Geometry: final body of the model. Coordinates: model frame, mm. A direction names the side the tool comes from. Give positions to 0.01 mm unless a question says otherwise; leave off trailing zeros. Loops run counter-clockwise (first coordinate to the right, second up) from the corner with the lowest first, then second, coordinate; pieces in that order, holes last. Notation, with made-up numbers: M 14.5,63.25 L 20.5,63.25 A21 ccw 20.5,75.25 Z; hole C 83.25,26.5 d8. An arc over 180 degrees is marked long. One line per question, with ' | ' between items. Start each with the question number.
from build123d import *

# Parameters (mm, degrees)
F0_W     = 25.5
F0_H     = 22
F0_R     = 3
F1_DEPTH = 2
F2_W     = 2
F2_H     = 5.4
F3_DEPTH = 25
F2_H_2   = 11.2
F4_DEPTH = 22.5
F5_R     = 2
F6_R     = 5
F7_DEPTH = 1.42
F8_R     = 1.25
F9_DEPTH = 2


with BuildPart() as f1:
    # F0 (on Top) → F1 (new body)
    with BuildSketch(Plane.XY):
        Rectangle(F0_W, F0_H)
        Circle(F0_R, mode=Mode.SUBTRACT)
    extrude(amount=F1_DEPTH)

    # F2 (on face) → F3 (join)
    with BuildSketch(Plane.XY.offset(2)):
        with Locations((-11.75, 8.3)):
            Rectangle(F2_W, F2_H)
        with Locations((11.75, 8.3)):
            Rectangle(F2_W, F2_H)
        with Locations((11.75, -8.3)):
            Rectangle(F2_W, F2_H)
        with Locations((-11.75, -8.3)):
            Rectangle(F2_W, F2_H)
    extrude(amount=F3_DEPTH)

    # F2 (on face) → F4 (join)
    with BuildSketch(Plane.XY.offset(2)):
        with Locations((11.75, 0)):
            Rectangle(F2_W, F2_H_2)
        with Locations((-11.75, 0)):
            Rectangle(F2_W, F2_H_2)
    extrude(amount=F4_DEPTH)

    # F5
    f5_edges = [f1.edges().sort_by_distance(p)[0] for p in [
        (12.75, 0, 0),
        (-12.75, 0, 0),
    ]]
    fillet(f5_edges, radius=F5_R)

    # F6 (on face) → F7 (join)
    with BuildSketch(Plane.XY.offset(24.5)):
        Polygon((10.75, -5.6), (12.75, -5.6), (12.75, 5.6), (10.75, 5.6), (10.75, 11), (-10.75, 11), (-10.75, 5.6), (-12.75, 5.6), (-12.75, -5.6), (-10.75, -5.6), (-10.75, -11), (10.75, -11), align=None)
        Circle(F6_R, mode=Mode.SUBTRACT)
    extrude(amount=F7_DEPTH)

    # F8 (on face) → F9 (cut, through all)
    with BuildSketch(Plane.YZ.offset(12.75)):
        with Locations((-6.1, 22.1)):
            Circle(F8_R)
        with Locations((6.092, 7.2918)):
            Circle(F8_R)
    extrude(amount=-F9_DEPTH, mode=Mode.SUBTRACT)


solid = f1.part
Q1. Contact query for flat-ended pins moving along their axis: pin 1 (11 mm diameter, centred on x = 3, y = -2.5, fed in from +Z); pin 2 (1.5 mm diameter, centred on y = -6.1, z = 22.1, fed in from +X); pin 3 (9.5 mm diameter, centred on x = 0, y = 0, fed in from +Z). Output: stop coordinate, or through.
Q2. Section A-A, the plane z = 22.1. Output: boundary loops of the cut face in (x, y), plus the area to 3 significant figures.
Q3. Section B-B, the plane x = -5.5. Output: boundary loops of the cut face in (y, z), plus the area to 3 significant figures.
Q4. Material intervals for L1, parallel to Y at x = 0, z = 1.5; L2, parallel to Z at x = 1, y = 8.75; L3, parallel to X at y = 6, z = 14.75, sorted ascending.
Q5. Draft query along X for faces 4 (the flat face through (-10.75, 0, 13)), 5 (the flat face through (12.75, 0, 14)), 6 (the flat face through (2, 3, 2)), 7 (the flat face through (11, -11, 13)). Return one class per face: released by +X, released by -X, zero draft, split by the parting line, or undercut.
Q6. Section D-D, the plane x = 0. Output: boundary loops of the cut face in (y, z).
Q7. Set-up query: faces 1 (the flat face through (5, 3, 24.5)), 2 (the flat face through (-10.75, -8.3, 26.5)), 3 (the flat face through (-11.8, 5.6, 26.5)). Return all of +Z, -Z, +X, -X, +Y, -Y with unobstructed straight access to the full face (end or side cutting, diameter ignored); none if empty.
Q8. Section C-C, the plane y = 0. Output: boundary loops of the cut face in (x, z), plus the area to 3 significant figures.
Model answer:
1) pin 1: stops at z = 25.92 | pin 2: stops at x = -10.75 | pin 3: stops at z = 2
2) outline: M -12.75,-11 L -10.75,-11 L -10.75,11 L -12.75,11 Z; M 10.75,-11 L 12.75,-11 L 12.75,-7.35 L 10.75,-7.35 Z; M 10.75,-4.85 L 12.75,-4.85 L 12.75,11 L 10.75,11 Z | area: 83.0 mm^2
3) outline: M -11,0 L 11,0 L 11,2 L -11,2 Z; M -11,24.5 L 11,24.5 L 11,25.92 L -11,25.92 Z | area: 75.2 mm^2
4) L1: y = -11 to -3, 3 to 11 | L2: z = 0 to 2, 24.5 to 25.92 | L3: x = -12.75 to -10.75, 10.75 to 12.75
5) face 4: undercut | face 5: released by +X | face 6: undercut | face 7: zero draft
6) outline: M -11,0 L -3,0 L -3,2 L -11,2 Z; M -11,24.5 L -5,24.5 L -5,25.92 L -11,25.92 Z; M 3,0 L 11,0 L 11,2 L 3,2 Z; M 5,24.5 L 11,24.5 L 11,25.92 L 5,25.92 Z
7) face 1: +Y, -Y | face 2: +Z, +Y, -Y | face 3: +Z, +X, -X
8) outline: M -12.75,2 A2 ccw -10.75,0 L -3,0 L -3,2 L -10.75,2 L -10.75,24.5 L -5,24.5 L -5,25.92 L -12.75,25.92 Z; M 3,0 L 10.75,0 A2 ccw 12.75,2 L 12.75,25.92 L 5,25.92 L 5,24.5 L 10.75,24.5 L 10.75,2 L 3,2 Z | area: 149 mm^2
